Part model, mm, in its own coordinate system. Round coordinates to 2 decimals unless told otherwise and drop trailing zeros. Loops run counter-clockwise (first coordinate to the right, second up) from the corner with the lowest first, then second, coordinate; pieces in that order, holes last. Notation, with made-up numbers: (19, -40) - (43, -40) arc R30 cw to (43, -12) - close; hole circle Ø4 at (25, 61). An arc over 180 degrees is marked (long way). Write each question's results on one line, items separated by ' | '. Start each with the question number.
(1) Cut at A-A, the plane x = 0. List the corners of the cut face in (y, z), then the cut area to 3 significant figures.
(2) Flat gauge pins, fed straight in: P1, Ø5, axis at x = -3.5, z = -1.5, coming from the +Y side; P2, Ø12, axis at x = 7, y = 24.5, coming from the +Z side; P3, Ø6, axis at y = 13, z = 3.5, coming from the -X side. Where does each tip first touch, or does it go through?
(3) Mould opens along X. For faces 1 (the face through (0, -0.152, 0)), 2 (the face through (-2.849, 14.103, -9.047)), 3 (the face through (-2.94, 14.103, -9.337)) say: released by +X, released by -X, zero draft, split by the parting line, or undercut.
(4) Drill centre lines: L1, parallel to Y at x = 5, z = -5.25; L2, parallel to X at y = 13.5, z = -3.75; L3, parallel to X at y = 5.25, z = 3.75. Where is each one in solid material? Low to high.
(5) Cut at C-C, the plane y = 14. List the corners of the cut face in (x, z).
(6) Cut at D-D, the plane y = 2.5. List the corners of the cut face in (x, z), then the cut area to 3 significant figures.
(7) Cut at B-B, the plane z = 0. List the corners of the cut face in (x, y).
Autodesk Inventor part; units mm, degrees
ref_plane "YZ Plane" through (0, 0, 0) normal (1, 0, 0) x (0, 1, 0)
ref_plane "XZ Plane" through (0, 0, 0) normal (0, 1, 0) x (-1, 0, 0)
ref_plane "XY Plane" through (0, 0, 0) normal (0, 0, 1) x (1, 0, 0)
sketch "Sketch1" plane through (0, 0, 0) normal (0, 0, 1) x (1, 0, 0)
  line L0 (0, 0) -> (8.4667, 0) construction
  arc A0 (8.4667, -0.1519) -> (8.4667, 0.1519) centre (8.4667, 0) ccw
  line L1 (8.4667, -0.1519) -> (0, -0.1519)
  line L2 (0, -0.1519) -> (0, 0)
  line L3 (8.4667, 0.1519) -> (0, 0.1519)
  line L4 (0, 0.1519) -> (0, 0)
  dimension "d0" = 8.4667
  dimension "d1" = 0.3037
  dimension "d2" = 8.4667
  dimension "d3" = 8.4667
revolve "bace" add sketch "Sketch1" angle 360 about axis through (0, 0.1519, 0) along (0, -1, 0)
sketch "Sketch2" plane through (0, 0, 0) normal (1, 0, 0) x (0, 1, 0)
  line L0 (0.1519, 8.4667) -> (0.1519, -8.4667)
  line L1 (0.1519, 0) -> (27.6685, 0)
  line L2 (27.6685, 0) -> (27.6685, -11.0747)
  line L3 (27.6685, -11.0747) -> (0.1519, -8.4667)
  line L4 (27.6685, -11.0747) -> (27.6685, -10.7709)
  line L5 (27.6685, -10.7709) -> (0.1519, -8.1629)
  line L6 (0.1519, -8.4667) -> (0.1519, -8.1629)
  point P0 (0, 0)
  dimension "d5" = 27.5167
  dimension "d6" = 0.3037
  dimension "d7" = 0.3037
revolve "walls" add sketch "Sketch2" angle 360 about axis through (0, 0.1519, 0) along (0, 1, 0) contours L5 L2 L3 L0
sketch "Sketch3" plane through (0, 0, 0) normal (0, 0, 1) x (1, 0, 0)
  line L0 (8.1629, 0.1519) -> (10.7709, 27.6685)
  line L1 (10.7709, 27.6685) -> (11.0747, 27.6685) construction
  line L2 (11.0747, 27.6685) -> (8.4667, 0.1519)
  line L3 (-11.0747, 27.6685) -> (11.0747, 27.6685)
  arc A0 (11.0747, 27.6685) -> (10.7709, 27.6685) centre (10.9228, 27.6685) ccw
  line L4 (0, -5.7418) -> (0, 33.3874)
  point P0 (0, 0)
  dimension "d10" = 0.1519
revolve "Revolution3" add sketch "Sketch3" angle 360 about axis through (0, -10, 0) along (0, 1, 0)
equation "\"d2\" = d0"
equation "\"d3\" = d0"
equation "\"d6\" = d1"
equation "\"d10\" = 0.5 * d1"
properties part number "trash bin 13 inches not demanding"
A:
1) outline: (-0.15, -8.47) arc R0.15 ccw to (0.15, -8.47) - (27.67, -11.07) arc R0.15 ccw to (27.67, -10.77) - (0.15, -8.16) - (0.15, 8.16) - (27.67, 10.77) arc R0.15 ccw to (27.67, 11.07) - (0.15, 8.47) arc R0.15 ccw to (-0.15, 8.47) - close | area: 22.0 mm2
2) P1: y = 0.15 | P2: z = 10.91 | P3: x = -9.79
3) face 1: zero draft | face 2: undercut | face 3: split by the parting line
4) L1: -0.15 to 0.15 | L2: -8.98 to -8.65, 8.65 to 8.98 | L3: -8.13 to -7.79, 7.79 to 8.13
5) outline: circle Ø19.56 at (0, 0); hole circle Ø18.95 at (0, 0)
6) outline: circle Ø17.38 at (0, 0); hole circle Ø16.77 at (0, 0) | area: 16.3 mm2
7) outline: (-11.07, 27.67) - (-8.47, 0.15) arc R0.15 ccw to (-8.47, -0.15) - (8.47, -0.15) arc R0.15 ccw to (8.47, 0.15) - (11.07, 27.67) arc R0.15 ccw to (10.77, 27.67) - (8.16, 0.15) - (-8.16, 0.15) - (-10.77, 27.67) arc R0.15 ccw to start
